Work out the finished part from the listing and answer in its coordinate system (mm). A direction names the side the tool comes from. Round coordinates to 2 decimals unless told otherwise and drop trailing zeros. Order: outer loops, then holes, each group sorted by start corner. A loop starts at its lowest first (then second) coordinate and runs counter-clockwise, first axis right, second up. Notation, with made-up numbers: (17.25, 3.5) - (34.25, 3.5) arc R23 cw to (34.25, 31.5) - close; hole circle Ø9 at (86, 57.5). An arc over 180 degrees is marked (long way). Use CSV: the item, a comma, the result in double quotes.
from build123d import *

# Parameters (mm, degrees)
SKETCH_1_W          = 120
SKETCH_1_H          = 120
SKETCH_1_R          = 3
SKETCH_1_R_2        = 2
SKETCH_1_R_3        = 15
EXTRUDE_1_DEPTH     = 3
CUT_EXTRUDE_1_DEPTH = 85.905830189
FILLET_1_R          = 10
FILLET_2_R          = 5
SKETCH_4_R          = 1.5
CUT_EXTRUDE_2_DEPTH = 85.905830189


with BuildPart() as part:
    # Эскиз1 → Бобышка-Вытянуть1 (new body)
    with BuildSketch(Plane(origin=(0, 0, 0), x_dir=(1, 0, 0), z_dir=(0, 1, 0))):
        Rectangle(SKETCH_1_W, SKETCH_1_H)
        with Locations(Location((0, 0, 0), (0, 0, 270))):
            Circle(SKETCH_1_R, mode=Mode.SUBTRACT)
        with Locations(Location((-48, 0, 0), (0, 0, 270))):
            Circle(SKETCH_1_R_2, mode=Mode.SUBTRACT)
        with Locations(Location((48, 0, 0), (0, 0, 90))):
            Circle(SKETCH_1_R_2, mode=Mode.SUBTRACT)
        with Locations(Location((0, 30, 0), (0, 0, 270))):
            Circle(SKETCH_1_R_3, mode=Mode.SUBTRACT)
    extrude(amount=EXTRUDE_1_DEPTH)

    # Эскиз3 → Вырез-Вытянуть1 (cut, through all)
    with BuildSketch(Plane(origin=(0, 3, 0), x_dir=(1, 0, 0), z_dir=(0, 1, 0))):
        Polygon((-60, 60), (-45, 60), (-45, 50), (-50, 50), (-50, 45), (-60, 45), align=None)
        Polygon((60, 45), (60, 60), (45, 60), (45, 50), (50, 50), (50, 45), align=None)
        Polygon((60, -60), (45, -60), (45, -50), (50, -50), (50, -45), (60, -45), align=None)
        Polygon((-60, -45), (-60, -60), (-45, -60), (-45, -50), (-50, -50), (-50, -45), align=None)
    extrude(amount=-CUT_EXTRUDE_1_DEPTH, mode=Mode.SUBTRACT)

    # Скругление1
    # the kernel refuses this fillet: 10 mm, written as the material it takes off along each edge
    with BuildSketch(Plane(origin=(50, 15.5, -50), x_dir=(0, 0, 1), z_dir=(0, -1, 0)), Plane(origin=(50, 15.5, 50), x_dir=(-1, 0, 0), z_dir=(0, -1, 0)), Plane(origin=(-50, 15.5, 50), x_dir=(0, 0, -1), z_dir=(0, -1, 0)), Plane(origin=(-50, 15.5, -50), x_dir=(1, 0, 0), z_dir=(0, -1, 0))) as fillet_1_piece_1:
        with BuildLine():
            CenterArc((9.114378278, 9.114378278), FILLET_1_R, 204.295188945, 41.409622109)
            Line((0, 5), (0, 0))
            Line((0, 0), (5, 0))
        make_face()
    extrude(amount=28, mode=Mode.SUBTRACT)

    # Скругление2
    fillet_2_edges = [part.edges().sort_by_distance(p)[0] for p in [
        (-60, 1.5, 45),
        (-45, 1.5, 60),
        (60, 1.5, 45),
        (45, 1.5, 60),
        (60, 1.5, -45),
        (45, 1.5, -60),
        (-60, 1.5, -45),
        (-45, 1.5, -60),
    ]]
    fillet(fillet_2_edges, radius=FILLET_2_R)

    # Эскиз4 → Вырез-Вытянуть2 (cut, through all)
    with BuildSketch(Plane(origin=(0, 3, 0), x_dir=(1, 0, 0), z_dir=(0, 1, 0))):
        with Locations(Location((0, 55, 0), (0, 0, 270))):
            Circle(SKETCH_4_R)
        with Locations(Location((18, 55, 0), (0, 0, 270))):
            Circle(SKETCH_4_R)
        with Locations(Location((36, 55, 0), (0, 0, 270))):
            Circle(SKETCH_4_R)
        with Locations(Location((-18, 55, 0), (0, 0, 270))):
            Circle(SKETCH_4_R)
        with Locations(Location((-36, 55, 0), (0, 0, 270))):
            Circle(SKETCH_4_R)
        with Locations(Location((55, 0, 0), (0, 0, 270))):
            Circle(SKETCH_4_R)
        with Locations(Location((55, -18, 0), (0, 0, 270))):
            Circle(SKETCH_4_R)
        with Locations(Location((55, -36, 0), (0, 0, 270))):
            Circle(SKETCH_4_R)
        with Locations(Location((55, 18, 0), (0, 0, 270))):
            Circle(SKETCH_4_R)
        with Locations(Location((55, 36, 0), (0, 0, 270))):
            Circle(SKETCH_4_R)
        with Locations(Location((0, -55, 0), (0, 0, 270))):
            Circle(SKETCH_4_R)
        with Locations(Location((-18, -55, 0), (0, 0, 270))):
            Circle(SKETCH_4_R)
        with Locations(Location((-36, -55, 0), (0, 0, 270))):
            Circle(SKETCH_4_R)
        with Locations(Location((18, -55, 0), (0, 0, 270))):
            Circle(SKETCH_4_R)
        with Locations(Location((36, -55, 0), (0, 0, 270))):
            Circle(SKETCH_4_R)
        with Locations(Location((-55, 0, 0), (0, 0, 270))):
            Circle(SKETCH_4_R)
        with Locations(Location((-55, 18, 0), (0, 0, 270))):
            Circle(SKETCH_4_R)
        with Locations(Location((-55, 36, 0), (0, 0, 270))):
            Circle(SKETCH_4_R)
        with Locations(Location((-55, -18, 0), (0, 0, 270))):
            Circle(SKETCH_4_R)
        with Locations(Location((-55, -36, 0), (0, 0, 270))):
            Circle(SKETCH_4_R)
    extrude(amount=-CUT_EXTRUDE_2_DEPTH, mode=Mode.SUBTRACT)


solid = part.part
(1) Find section D-D (y = 1.85). State how many separate pieces and enclosed holes the cut face has, and give its area (3 significant figures).
Findings below:
separate pieces,"1"
enclosed holes,"24"
area,"12,600 mm²"
(2) For faces 4 (the flat face through (-45, 2, -53)), 5 (the flat face through (45, 2, 53)), 6 (the cylindrical face through (0.45, 1.52, 56.43)), 7 (the flat face through (52, 2, -45)), 8 (the flat face through (-52, 2, 45)), determine the directions among +Z, -Z, +X, -X, +Y, -Y from which every point of the face is accessible in a straight line to the end or side of a thin tool.
Findings below:
face 4,"-Z, -X, +Y, -Y"
face 5,"+Z, +X, +Y, -Y"
face 6,"+Y, -Y"
face 7,"-Z, +X, +Y, -Y"
face 8,"+Z, -X, +Y, -Y"
(3) Find section C-C (x = -48). Determine the outline of the cut face in (y, z), and give its area (3 significant figures).
Findings below:
outline,"(0, -47.91) - (3, -47.91) - (3, -2) - (0, -2) - close; (0, 2) - (3, 2) - (3, 47.91) - (0, 47.91) - close"
area,"275 mm²"
(4) Find section A-A (z = -30). Determine the outline of the cut face in (x, y).
Findings below:
outline,"(-60, 0) - (-15, 0) - (-15, 3) - (-60, 3) - close; (15, 0) - (60, 0) - (60, 3) - (15, 3) - close"
(5) The mould has two halves that part along X. Classify faces 1 (the flat face through (-45, 2, 53)), 2 (the cylindrical face through (54.1, 1.5, -37.2)), 3 (the flat face through (-1, 3, 12)): released by +X, released by -X, zero draft, split by the parting line, or undercut.
Findings below:
face 1,"released by -X"
face 2,"undercut"
face 3,"zero draft"
(6) Find the intervals of material crossed by L1, parallel to X at y = 1.7, z = 36; L2, parallel to X at y = 1.45, z = 55; L3, parallel to X at y = 1.15, z = 0, in increasing order. Write a range as from..to.
Findings below:
L1,"x = -60..-56.5, -53.5..53.5, 56.5..60"
L2,"x = -45..-37.5, -34.5..-19.5, -16.5..-1.5, 1.5..16.5, 19.5..34.5, 37.5..45"
L3,"x = -60..-56.5, -53.5..-50, -46..-3, 3..46, 50..53.5, 56.5..60"
(7) Find section B-B (x = 18). Determine the outline of the cut face in (y, z), and give its area (3 significant figures).
Findings below:
outline,"(0, -60) - (3, -60) - (3, -56.5) - (0, -56.5) - close; (0, -53.5) - (3, -53.5) - (3, 53.5) - (0, 53.5) - close; (0, 56.5) - (3, 56.5) - (3, 60) - (0, 60) - close"
area,"342 mm²"
(8) Each of these flat-tipped pins is pushed along its axis until it touches: pin 1 (0.9 mm diameter, centred on x = 52, y = 2, fed in from +Z); pin 2 (1.8 mm diameter, centred on x = -55, z = -36, fed in from -Y); pin 3 (0.9 mm diameter, centred on y = 1.5, z = -51.5, fed in from +X); pin 4 (0.9 mm diameter, centred on y = 2, z = -52, fed in from -X). Where does it stop, or does it pass through?
Findings below:
pin 1,"stops at z = 45"
pin 2,"passes through"
pin 3,"stops at x = 45"
pin 4,"stops at x = -45"
